Print and shaded views of the part. All mm, measured from the part's lowest x, y and z. Coordinates: 2 decimals unless noted, no trailing zeros. Order: outer loops, then holes, each group sorted by start corner. A loop starts at its lowest first (then second) coordinate and runs counter-clockwise, first axis right, second up. Notation, with made-up numbers: (-37.75, 30.5) -> (-8.75, 30.5) arc R28 ccw to (-8.75, 69.5) -> close; hole circle Ø10 at (20.5, 35). An arc over 180 degrees is marked (long way). Write item = value, one per line. Start each with the question number.
Q1. Cut at A-A, the plane z = 209.5. List the corners of the cut face in (x, y).
Q2. Cut at D-D, the plane x = 142. List the corners of the cut face in (y, z), plus the area to 4 significant figures.
Q3. Cut at C-C, the plane z = 243. List the corners of the cut face in (x, y), plus the area to 4 significant figures.
Q4. Wall check: line 1 (X direction, y = 1.7, z = 183); line 2 (Z direction, x = 142, y = 3.45); line 3 (Z direction, x = 86.5, y = 2.7). Give the ranges that are in metal, low to high. Write a range as from..to.
Q5. Cut at B-B, the plane x = 59. List the corners of the cut face in (y, z).
Q6. Flat gauge pins, fed straight in: pin 1 (4 mm diameter, centred on x = 139, y = 3.5, fed in from -Z); pin 2 (2.5 mm diameter, centred on y = 1.5, z = 258, fed in from +X); pin 3 (1.5 mm diameter, centred on y = 4, z = 85.5, fed in from -X); pin 4 (1.5 mm diameter, centred on x = 92.5, y = 2, fed in from -Z). Where does each tip first touch, or does it go through?
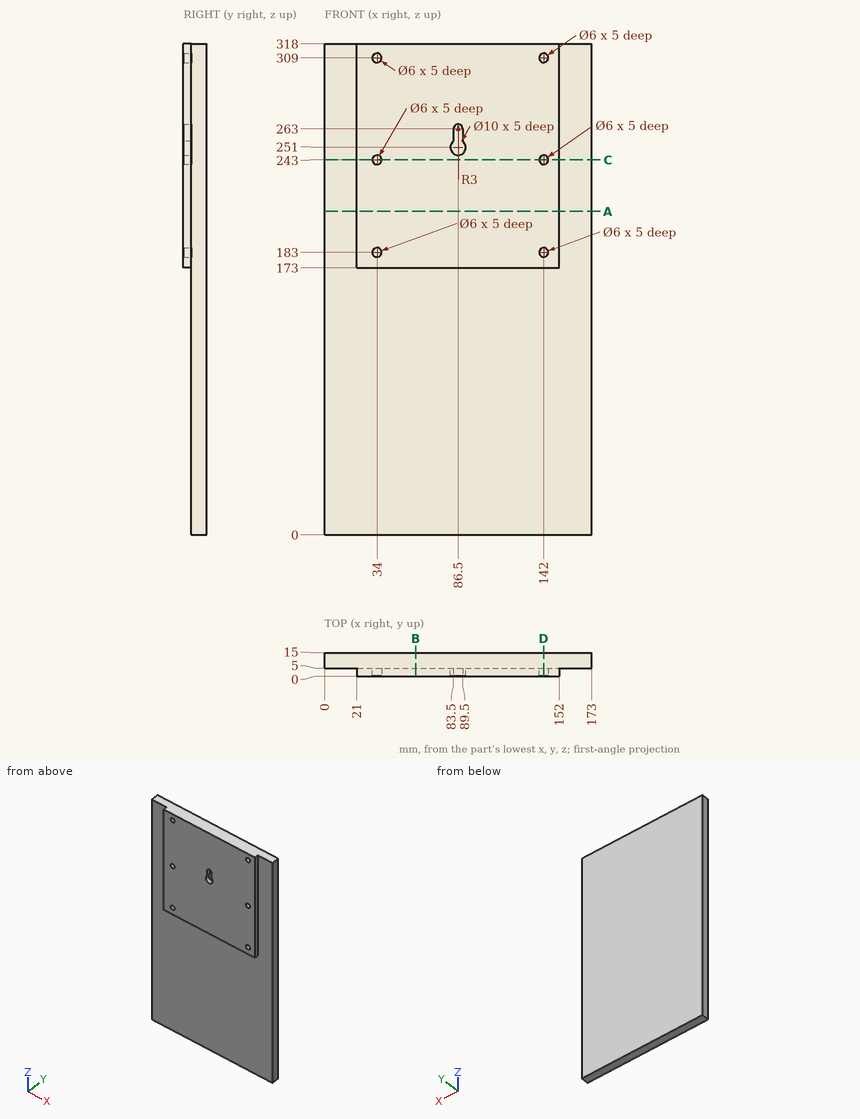
Here are the results:
q1.outline = (0, 5) -> (21, 5) -> (21, 0) -> (152, 0) -> (152, 5) -> (173, 5) -> (173, 15) -> (0, 15) -> close
q2.outline = (0, 173) -> (5, 173) -> (5, 0) -> (15, 0) -> (15, 318) -> (0, 318) -> (0, 312) -> (5, 312) -> (5, 306) -> (0, 306) -> (0, 246) -> (5, 246) -> (5, 240) -> (0, 240) -> (0, 186) -> (5, 186) -> (5, 180) -> (0, 180) -> close
q2.area = 3,815 mm²
q3.outline = (0, 5) -> (21, 5) -> (21, 0) -> (31, 0) -> (31, 5) -> (37, 5) -> (37, 0) -> (139, 0) -> (139, 5) -> (145, 5) -> (145, 0) -> (152, 0) -> (152, 5) -> (173, 5) -> (173, 15) -> (0, 15) -> close
q3.area = 2,325 mm²
q4.line_1 = 21..31, 37..139, 145..152
q4.line_2 = 173..180, 186..240, 246..306, 312..318
q4.line_3 = 173..246, 266..318
q5.outline = (0, 173) -> (5, 173) -> (5, 0) -> (15, 0) -> (15, 318) -> (0, 318) -> close
q6.pin_1 = 0
q6.pin_2 = 152
q6.pin_3 = through
q6.pin_4 = 173
